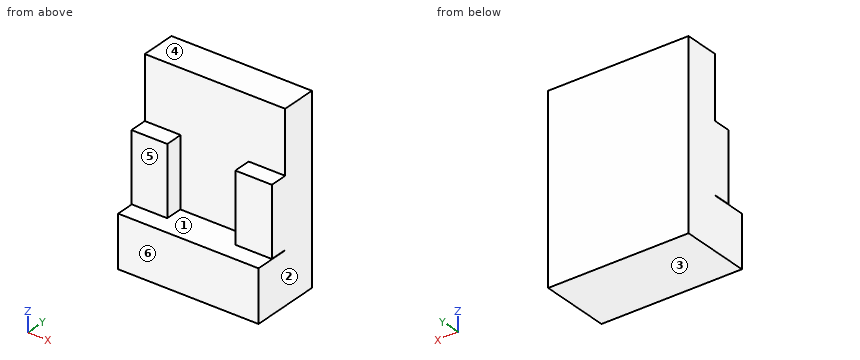
```python
from build123d import *

# Parameters (mm, degrees)
F0_W     = 21.0800419182
F0_H     = 51.430279389
F0_W_2   = 21.0800442
F1_DEPTH = 50.8
F2_W     = 26.432774961
F2_H     = 49.8542264104
F3_DEPTH = 12.7
F4_W     = 102.5741808116
F4_H     = 37.7440936863
F5_DEPTH = 25.4
F6_DEPTH = 25.4
F7_DEPTH = 25.4


with BuildPart() as f1:
    # F0 (on Front) → F1 (new body)
    with BuildSketch(Plane.XZ):
        with Locations((-39.4168676153, -2.9509169981)):
            Rectangle(F0_W, F0_H)
        with Locations((41.1030893256, -2.9509169981)):
            Rectangle(F0_W_2, F0_H)
        Polygon((51.6431114256, 66.6497073153), (-49.9568885744, 66.6497073153), (-49.9568885744, 22.7642226964), (-28.8768466562, 22.7642226964), (-28.8768466562, -28.6660566926), (30.5630672256, -28.6660566926), (30.5630672256, 22.7642226964), (51.6431114256, 22.7642226964), align=None)
        Polygon((-28.8768466562, -28.6660566926), (-49.9568885744, -28.6660566926), (-49.9568885744, -65.8065884391), (51.6431114256, -65.8065884391), (51.6431114256, -28.6660566926), (30.5630672256, -28.6660566926), align=None)
    extrude(amount=-F1_DEPTH)

    # F2 (on Front) → F3 (cut)
    with BuildSketch(Plane.XZ):
        with Locations((38.4267239451, -3.2813642174)):
            Rectangle(F2_W, F2_H)
        Polygon((-50.4875965416, -28.2084774226), (-50.1530058682, -28.2084774226), (-24.0548325416, -28.2084774226), (-24.0548325416, 21.6457535774), (-50.4875965416, 21.6457535774), align=None)
    extrude(amount=-F3_DEPTH, mode=Mode.SUBTRACT)

    # F4 (on Front) → F5 (join)
    with BuildSketch(Plane.XZ):
        with Locations((0.5936603993, -47.2895335406)):
            Rectangle(F4_W, F4_H)
    extrude(amount=F5_DEPTH)

    # F6 (cut): a face of the model
    f6_faces = [f1.faces().sort_by_distance(p)[0] for p in [
        (0.7506624664, 0, 27.4054577125),
    ]]
    extrude(f6_faces, amount=-F6_DEPTH, mode=Mode.SUBTRACT)

    # F7 (cut): a face of the model
    f7_faces = [f1.faces().sort_by_distance(p)[0] for p in [
        (0.5936603993, -25.4, -47.2895335406),
    ]]
    extrude(f7_faces, amount=-F7_DEPTH, mode=Mode.SUBTRACT)


solid = f1.part
```
Could you check a few things on this model? Use its own coordinates, in mm. Face numbers are marked on the shaded views. A direction names the side the tool comes from. Coordinates: 2 decimals unless noted, no trailing zeros. Order: outer loops, then holes, each group sorted by start corner. A loop starts at its lowest first (then second) coordinate and runs counter-clockwise, first axis right, second up. Notation, with made-up numbers: M -37.5,-19.5 L 5.5,-19.5 A29 cw 5.5,13.5 Z; hole C -37,64.25 d3. An arc over 180 degrees is marked long. Use a Markdown table: item, result. Add a question column.
Q1. I want a section at D-D on z = 57.5. List the corners of the cut face in (x, y) for me, then the cut area to 3 significant figures.
Q2. I want a section at C-C on x = -29. List the corners of the cut face in (y, z) for me, then the cut area to 3 significant figures.
Q3. I want a section at B-B on x = 4. List the corners of the cut face in (y, z) for me, then the cut area to 3 significant figures.
Q4. Which directions (+Z, -Z, +X, -X, +Y, -Y) give clear straight access to the entire face, cutting with the end or side of a thin tool? Please do the marked faces 5 and 6.
Q5. I'm going to push flat-ended pins straight in: pin 1 (3 mm diameter, centred on x = 18, z = 21, fed in from -Y); pin 2 (7.5 mm diameter, centred on x = -14.5, y = 15.5, fed in from +Z); pin 3 (3 mm diameter, centred on x = 32, y = 23.5, fed in from +Z). Where does each tip first touch, or does it pass through?
Q6. If I drill on L1, parallel to X at y = 14.5, z = 2.5; L2, parallel to Y at x = 24, z = 61; L3, parallel to Z at x = 7.5, y = 22, over which ranges is the centre line in solid material (lowest first)?
Q7. We'd pull the mould along Z, two halves only. Please class the marked faces 1, 2, 3 and 4: pulls with the +Z half, pulls with the -Z half, needs draft (parallel to the pull), parting line crosses it, or undercut.
Q8. I want a section at A-A on z = -16. List the corners of the cut face in (x, y) for me.
Checked values:
| question | item | result |
|---|---|---|
| 1 | outline | M -49.96,25.4 L 51.64,25.4 L 51.64,50.8 L -49.96,50.8 Z |
| 1 | area | 2,580 mm² |
| 2 | outline | M 0,-65.81 L 50.8,-65.81 L 50.8,66.65 L 25.4,66.65 L 25.4,21.65 L 12.7,21.65 L 12.7,-28.21 L 25.4,-28.21 L 25.4,-28.42 L 0,-28.42 Z |
| 2 | area | 4,950 mm² |
| 3 | outline | M 0,-65.81 L 50.8,-65.81 L 50.8,66.65 L 25.4,66.65 L 25.4,-28.42 L 0,-28.42 Z |
| 3 | area | 4,310 mm² |
| 4 | face 5 | +Z, +X, -X, -Y |
| 4 | face 6 | +Z, -Z, +X, -X, -Y |
| 5 | pin 1 | y = 25.4 |
| 5 | pin 2 | z = -28.42 |
| 5 | pin 3 | z = 21.65 |
| 6 | L1 | -49.96 to -24.05, 25.21 to 51.64 |
| 6 | L2 | 25.4 to 50.8 |
| 6 | L3 | -65.81 to -28.42 |
| 7 | face 1 | undercut |
| 7 | face 2 | needs draft |
| 7 | face 3 | pulls with the -Z half |
| 7 | face 4 | pulls with the +Z half |
| 8 | outline | M -49.96,12.7 L -24.05,12.7 L -24.05,25.4 L 25.21,25.4 L 25.21,12.7 L 51.64,12.7 L 51.64,50.8 L -49.96,50.8 Z |
